from build123d import *

# Parameters (mm, degrees)
BOSS_EXTRUDE1_DEPTH = 100


with BuildPart() as part:
    # Sketch1 → Boss-Extrude1 (new body)
    with BuildSketch(Plane(origin=(0, 0, 0), x_dir=(1, 0, 0), z_dir=(0, 1, 0))):
        with BuildLine():
            Line((-20, 4), (-20, 16))
            ThreePointArc((-20, 16), (-18.828427125, 18.828427125), (-16, 20))
            Line((-16, 20), (-4, 20))
            Line((-4, 20), (-4, 15.5))
            Line((-4, 15.5), (-11.25, 15.5))
            Line((-11.25, 15.5), (-11.25, 14))
            Line((-11.25, 14), (-5, 7.75))
            Line((-5, 7.75), (0, 7.75))
            Line((0, 7.75), (5, 7.75))
            Line((5, 7.75), (11.25, 14))
            Line((11.25, 14), (11.25, 15.5))
            Line((11.25, 15.5), (4, 15.5))
            Line((4, 15.5), (4, 20))
            Line((4, 20), (16, 20))
            ThreePointArc((16, 20), (18.828427125, 18.828427125), (20, 16))
            Line((20, 16), (20, 4))
            Line((20, 4), (15.5, 4))
            Line((15.5, 4), (15.5, 11.25))
            Line((15.5, 11.25), (14, 11.25))
            Line((14, 11.25), (7.75, 5))
            Line((7.75, 5), (7.75, 0))
            Line((7.75, 0), (7.75, -5))
            Line((7.75, -5), (14, -11.25))
            Line((14, -11.25), (15.5, -11.25))
            Line((15.5, -11.25), (15.5, -4))
            Line((15.5, -4), (20, -4))
            Line((20, -4), (20, -16))
            ThreePointArc((20, -16), (18.828427125, -18.828427125), (16, -20))
            Line((16, -20), (4, -20))
            Line((4, -20), (4, -15.5))
            Line((4, -15.5), (11.25, -15.5))
            Line((11.25, -15.5), (11.25, -14))
            Line((11.25, -14), (5, -7.75))
            Line((5, -7.75), (0, -7.75))
            Line((0, -7.75), (-5, -7.75))
            Line((-5, -7.75), (-11.25, -14))
            Line((-11.25, -14), (-11.25, -15.5))
            Line((-11.25, -15.5), (-4, -15.5))
            Line((-4, -15.5), (-4, -20))
            Line((-4, -20), (-16, -20))
            ThreePointArc((-16, -20), (-18.828427125, -18.828427125), (-20, -16))
            Line((-20, -16), (-20, -4))
            Line((-20, -4), (-15.5, -4))
            Line((-15.5, -4), (-15.5, -11.25))
            Line((-15.5, -11.25), (-14, -11.25))
            Line((-14, -11.25), (-7.75, -5))
            Line((-7.75, -5), (-7.75, 0))
            Line((-7.75, 0), (-7.75, 5))
            Line((-7.75, 5), (-14, 11.25))
            Line((-14, 11.25), (-15.5, 11.25))
            Line((-15.5, 11.25), (-15.5, 4))
            Line((-15.5, 4), (-20, 4))
        make_face()
        with BuildLine():
            Line((-18, 13.25), (-18, 16))
            ThreePointArc((-18, 16), (-17.414213562, 17.414213562), (-16, 18))
            Line((-16, 18), (-13.25, 18))
            Line((-13.25, 18), (-13.25, 13.957106781))
            Line((-13.25, 13.957106781), (-12.801776695, 13.508883476))
            Line((-12.801776695, 13.508883476), (-13.508883476, 12.801776695))
            Line((-13.508883476, 12.801776695), (-13.957106781, 13.25))
            Line((-13.957106781, 13.25), (-18, 13.25))
        make_face(mode=Mode.SUBTRACT)
        with BuildLine():
            Line((-12.448223305, 11.741116524), (-5.75, 5.042893219))
            Line((-5.75, 5.042893219), (-5.75, 2.90473751))
            Line((-5.75, 2.90473751), (-5.25, 2.90473751))
            Line((-5.25, 2.90473751), (-4.069705149, 2.90473751))
            ThreePointArc((-4.069705149, 2.90473751), (-3.535533906, 3.535533906), (-2.90473751, 4.069705149))
            Line((-2.90473751, 4.069705149), (-2.90473751, 5.25))
            Line((-2.90473751, 5.25), (-2.90473751, 5.75))
            Line((-2.90473751, 5.75), (-5.042893219, 5.75))
            Line((-5.042893219, 5.75), (-11.741116524, 12.448223305))
            Line((-11.741116524, 12.448223305), (-12.448223305, 11.741116524))
        make_face(mode=Mode.SUBTRACT)
        with BuildLine():
            Line((18, 13.25), (18, 16))
            ThreePointArc((18, 16), (17.414213562, 17.414213562), (16, 18))
            Line((16, 18), (13.25, 18))
            Line((13.25, 18), (13.25, 13.957106781))
            Line((13.25, 13.957106781), (12.801776695, 13.508883476))
            Line((12.801776695, 13.508883476), (13.508883476, 12.801776695))
            Line((13.508883476, 12.801776695), (13.957106781, 13.25))
            Line((13.957106781, 13.25), (18, 13.25))
        make_face(mode=Mode.SUBTRACT)
        with BuildLine():
            Line((5.75, 5.042893219), (5.75, 2.90473751))
            Line((5.75, 2.90473751), (5.25, 2.90473751))
            Line((5.25, 2.90473751), (4.069705149, 2.90473751))
            ThreePointArc((4.069705149, 2.90473751), (3.535533906, 3.535533906), (2.90473751, 4.069705149))
            Line((2.90473751, 4.069705149), (2.90473751, 5.25))
            Line((2.90473751, 5.25), (2.90473751, 5.75))
            Line((2.90473751, 5.75), (5.042893219, 5.75))
            Line((5.042893219, 5.75), (11.741116524, 12.448223305))
            Line((11.741116524, 12.448223305), (12.448223305, 11.741116524))
            Line((12.448223305, 11.741116524), (5.75, 5.042893219))
        make_face(mode=Mode.SUBTRACT)
        with BuildLine():
            Line((13.25, -18), (16, -18))
            ThreePointArc((16, -18), (17.414213562, -17.414213562), (18, -16))
            Line((18, -16), (18, -13.25))
            Line((18, -13.25), (13.957106781, -13.25))
            Line((13.957106781, -13.25), (13.508883476, -12.801776695))
            Line((13.508883476, -12.801776695), (12.801776695, -13.508883476))
            Line((12.801776695, -13.508883476), (13.25, -13.957106781))
            Line((13.25, -13.957106781), (13.25, -18))
        make_face(mode=Mode.SUBTRACT)
        with BuildLine():
            Line((5.042893219, -5.75), (2.90473751, -5.75))
            Line((2.90473751, -5.75), (2.90473751, -5.25))
            Line((2.90473751, -5.25), (2.90473751, -4.069705149))
            ThreePointArc((2.90473751, -4.069705149), (3.535533906, -3.535533906), (4.069705149, -2.90473751))
            Line((4.069705149, -2.90473751), (5.25, -2.90473751))
            Line((5.25, -2.90473751), (5.75, -2.90473751))
            Line((5.75, -2.90473751), (5.75, -5.042893219))
            Line((5.75, -5.042893219), (12.448223305, -11.741116524))
            Line((12.448223305, -11.741116524), (11.741116524, -12.448223305))
            Line((11.741116524, -12.448223305), (5.042893219, -5.75))
        make_face(mode=Mode.SUBTRACT)
        with BuildLine():
            Line((-18, -13.25), (-18, -16))
            ThreePointArc((-18, -16), (-17.414213562, -17.414213562), (-16, -18))
            Line((-16, -18), (-13.25, -18))
            Line((-13.25, -18), (-13.25, -13.957106781))
            Line((-13.25, -13.957106781), (-12.801776695, -13.508883476))
            Line((-12.801776695, -13.508883476), (-13.508883476, -12.801776695))
            Line((-13.508883476, -12.801776695), (-13.957106781, -13.25))
            Line((-13.957106781, -13.25), (-18, -13.25))
        make_face(mode=Mode.SUBTRACT)
        with BuildLine():
            Line((-5.75, -5.042893219), (-5.75, -2.90473751))
            Line((-5.75, -2.90473751), (-5.25, -2.90473751))
            Line((-5.25, -2.90473751), (-4.069705149, -2.90473751))
            ThreePointArc((-4.069705149, -2.90473751), (-3.535533906, -3.535533906), (-2.90473751, -4.069705149))
            Line((-2.90473751, -4.069705149), (-2.90473751, -5.25))
            Line((-2.90473751, -5.25), (-2.90473751, -5.75))
            Line((-2.90473751, -5.75), (-5.042893219, -5.75))
            Line((-5.042893219, -5.75), (-11.741116524, -12.448223305))
            Line((-11.741116524, -12.448223305), (-12.448223305, -11.741116524))
            Line((-12.448223305, -11.741116524), (-5.75, -5.042893219))
        make_face(mode=Mode.SUBTRACT)
        with BuildLine():
            ThreePointArc((-3.4, 0), (-2.404163056, 2.404163056), (0, 3.4))
            ThreePointArc((0, 3.4), (2.404163056, 2.404163056), (3.4, 0))
            ThreePointArc((3.4, 0), (2.404163056, -2.404163056), (0, -3.4))
            ThreePointArc((0, -3.4), (-2.404163056, -2.404163056), (-3.4, 0))
        make_face(mode=Mode.SUBTRACT)
    extrude(amount=BOSS_EXTRUDE1_DEPTH)


solid = part.part
Build history of the part. All positions in model axes, mm. A direction names the side the tool comes from. Round coordinates to 2 decimals unless told otherwise and drop trailing zeros. Write each loop counter-clockwise with the first axis right and the second up, starting at its lowest first coordinate (ties: lowest second). Pieces come first, ordered by that corner, then holes. Notation, with made-up numbers: M 17.25,59.25 L 54.25,59.25 A24 ccw 54.25,94.25 Z; hole C 0.25,87 d10. An arc over 180 degrees is marked long. Use CSV: the item, a comma, the result in double quotes.
1. Two-plate mould, pull along X, no slides. Class faces 3 (the face through (-18.859, 49.3, -18.797)), 4 (the face through (-5.75, 49, -4)), 5 (the face through (-4, 100, 0)): +X half, -X half, draft (parallel to the pull), parting line (faces both ways), or undercut.
Reply:
face 3,"-X half"
face 4,"undercut"
face 5,"draft"
2. Wall check: probe 1 along X at (y, z) = (23.5, 16); probe 2 along X at (y, z) = (77, -14); probe 3 along X at (y, z) = (88.5, -4.5). Give the ranges that are in metal, low to high. Write a range as from..to.
Reply:
probe 1,"x = -20..-18, -13.25..-4, 4..13.25, 18..20"
probe 2,"x = -20..-18, -13.25..-11.25, 11.25..13.25, 18..20"
probe 3,"x = -20..-15.5, -7.75..-5.75, -2.9..2.9, 5.75..7.75, 15.5..20"
3. Saw through at D-D (x = 17). Give the cut face in (y, z).
Reply:
outline,"M 0,-19.87 L 100,-19.87 L 100,-17.73 L 0,-17.73 Z; M 0,-13.25 L 100,-13.25 L 100,-4 L 0,-4 Z; M 0,4 L 100,4 L 100,13.25 L 0,13.25 Z; M 0,17.73 L 100,17.73 L 100,19.87 L 0,19.87 Z"
4. Saw through at A-A (z = 1.5). Give the cut face in (x, y).
Reply:
outline,"M -7.75,0 L -3.05,0 L -3.05,100 L -7.75,100 Z; M 3.05,0 L 7.75,0 L 7.75,100 L 3.05,100 Z"
5. Tool access for faces 1 (the face through (-18.797, 49.3, 18.859)), 2 (the face through (-8, 49, -15.5)): list every direction of +Z, -Z, +X, -X, +Y, -Y with a clear straight run to the whole face (end or side of a thin tool).
Reply:
face 1,"+Z, -X, +Y, -Y"
face 2,"+Y, -Y"
6. Flat gauge pins, fed straight in: pin 1 (5 mm diameter, centred on y = 45, z = -18, fed in from -X); pin 2 (1.3 mm diameter, centred on y = 30, z = 17, fed in from +X). Where does each tip first touch, or does it go through?
Reply:
pin 1,"stops at x = -20"
pin 2,"stops at x = 19.98"
7. Saw through at C-C (z = -9). Give the cut face in (x, y).
Reply:
outline,"M -20,0 L -15.5,0 L -15.5,100 L -20,100 Z; M -11.75,0 L -9.71,0 L -9.71,100 L -11.75,100 Z; M -8.29,0 L -6.25,0 L -6.25,100 L -8.29,100 Z; M 6.25,0 L 8.29,0 L 8.29,100 L 6.25,100 Z; M 9.71,0 L 11.75,0 L 11.75,100 L 9.71,100 Z; M 15.5,0 L 20,0 L 20,100 L 15.5,100 Z"
8. Saw through at B-B (x = -1). Give the cut face in (y, z), plus the area to 3 significant figures.
Reply:
outline,"M 0,-7.75 L 100,-7.75 L 100,-3.25 L 0,-3.25 Z; M 0,3.25 L 100,3.25 L 100,7.75 L 0,7.75 Z"
area,"900 mm²"
